Geometry check sheet. Reference: the model listing, model coordinates, mm. A direction names the side the tool comes from. Coordinates: 2 decimals unless noted, no trailing zeros. Order: outer loops, then holes, each group sorted by start corner. A loop starts at its lowest first (then second) coordinate and runs counter-clockwise, first axis right, second up. Notation, with made-up numbers: (31, 46.25) -> (61, 46.25) arc R21 cw to (61, 57.25) -> close; hole circle Ø3 at (5, 58). An arc over 180 degrees is marked (long way). Answer in a Markdown table with one row per item. Add a question column.
```python
from build123d import *


with BuildPart() as part:
    # Эскиз1 → Повернуть1 (revolve)
    with BuildSketch(Plane(origin=(0, 0, 0), x_dir=(0, 0, -1), z_dir=(1, 0, 0))):
        with BuildLine():
            Line((2.5, 16), (2.5, 9))
            Line((2.5, 9), (4, 9))
            Line((4, 9), (4, 8))
            Line((4, 8), (3, 8))
            Line((3, 8), (3, -0.5))
            ThreePointArc((3, -0.5), (2.707106781, -1.207106781), (2, -1.5))
            Line((2, -1.5), (1, -1.5))
            Line((1, -1.5), (1, 17))
            Line((1, 17), (1.5, 17))
            ThreePointArc((1.5, 17), (2.207106781, 16.707106781), (2.5, 16))
        make_face()
    revolve(axis=Axis((0, 0, 0), (0, 1, 0)))


solid = part.part
```
(1) Go/stop test with flat-tipped pins: P1, Ø2, axis at x = 3, y = 11.5, coming from the +Z side; P2, Ø1.5, axis at x = 0, y = 12.5, coming from the -Z side; P3, Ø1, axis at y = 0.5, z = 2.5, coming from the +X side. Record where each tip stops, or that it passes through.
(2) Cross-section at C-C (y = 14.25). Enter the section's corners in (x, z).
(3) Cross-section at D-D (y = 3.75). Enter the section's corners in (x, z), plus the area to 3 significant figures.
(4) Cross-section at A-A (z = 0). Enter the section's corners in (x, y), plus the area to 3 significant figures.
(5) Access from +Z, -Z, +X, -X, +Y, -Y to the whole of each face (thin tool, end or side, straight path). Record for faces 4 (the face through (2.44, 12.45, 0.54)), 5 (the face through (0, 4, 3)).
(6) Cross-section at B-B (x = 0). Enter the section's corners in (y, z).
(7) Mould release check, pull along Z, two halves, no side actions. Record for faces 1 (the face through (1, 8, 0)), 2 (the face through (3.905, 8.493, 0.867)), 3 (the face through (1, -1.5, -1)): +Z half, -Z half, draft (parallel to the pull), parting line (faces both ways), or undercut.
(8) Scan lines: line 1 along X through (y, z) = (11, 0); line 2 along Z through (x, y) = (0, 6.25). Record each from-to range of solid material in increasing order.
Checks:
| question | item | result |
|---|---|---|
| 1 | P1 | z = 1.5 |
| 1 | P2 | z = -2.5 |
| 1 | P3 | x = 2.24 |
| 2 | outline | circle Ø5 at (0, 0); hole circle Ø2 at (0, 0) |
| 3 | outline | circle Ø6 at (0, 0); hole circle Ø2 at (0, 0) |
| 3 | area | 25.1 mm² |
| 4 | outline | (-4, 8) -> (-3, 8) -> (-3, -0.5) arc R1 ccw to (-2, -1.5) -> (-1, -1.5) -> (-1, 17) -> (-1.5, 17) arc R1 ccw to (-2.5, 16) -> (-2.5, 9) -> (-4, 9) -> close; (1, -1.5) -> (2, -1.5) arc R1 ccw to (3, -0.5) -> (3, 8) -> (4, 8) -> (4, 9) -> (2.5, 9) -> (2.5, 16) arc R1 ccw to (1.5, 17) -> (1, 17) -> close |
| 4 | area | 67.1 mm² |
| 5 | face 4 | +Y |
| 5 | face 5 | -Y |
| 6 | outline | (-1.5, -2) arc R1 ccw to (-0.5, -3) -> (8, -3) -> (8, -4) -> (9, -4) -> (9, -2.5) -> (16, -2.5) arc R1 ccw to (17, -1.5) -> (17, -1) -> (-1.5, -1) -> close; (-1.5, 1) -> (17, 1) -> (17, 1.5) arc R1 ccw to (16, 2.5) -> (9, 2.5) -> (9, 4) -> (8, 4) -> (8, 3) -> (-0.5, 3) arc R1 ccw to (-1.5, 2) -> close |
| 7 | face 1 | undercut |
| 7 | face 2 | parting line |
| 7 | face 3 | draft |
| 8 | line 1 | -2.5 to -1, 1 to 2.5 |
| 8 | line 2 | -3 to -1, 1 to 3 |
